Job drawing, mm, ordinate dimensions from the low corner. One solid piece. Give positions to 0.01 mm unless a question says otherwise; leave off trailing zeros. Order: outer loops, then holes, each group sorted by start corner. A loop starts at its lowest first (then second) coordinate and runs counter-clockwise, first axis right, second up. Notation, with made-up numbers: (43, 68) -> (92, 68) arc R6 ccw to (92, 74) -> close; hole circle Ø10 at (37.5, 41). An arc over 180 degrees is marked (long way). Write item = value, one per line. Start each with the question number.
(1) Flat gauge pins, fed straight in: pin 1 (4 mm diameter, centred on x = 27, y = 51.875, fed in from -Z); pin 2 (1.5 mm diameter, centred on x = 12, z = 1.5, fed in from -Y); pin 3 (2.5 mm diameter, centred on x = 51.875, y = 27, fed in from -Z); pin 4 (1 mm diameter, centred on x = 6, z = 4.5, fed in from -Y). Where does each tip first touch, or does it go through?
(2) Saw through at A-A, the plane x = 27. List the corners of the cut face in (y, z) (3 decimals).
(3) Two-plate mould, pull along Y, no slides. Class the marked faces 1, 2 and 3: pulls with the +Y half, pulls with the -Y half, needs draft (parallel to the pull), parting line crosses it, or undercut.
(4) Probe line 1 along Y through (x, z) = (27, 5) (3 decimals); line 2 along X through (y, z) = (17, 8.5); line 3 along X through (y, z) = (20, 8). List the from-to ranges inside material, lowest first. Write a range as from..to.
(5) Saw through at B-B, the plane z = 4.5. List the corners of the cut face in (x, y) (3 decimals), then the cut area to 3 significant figures.
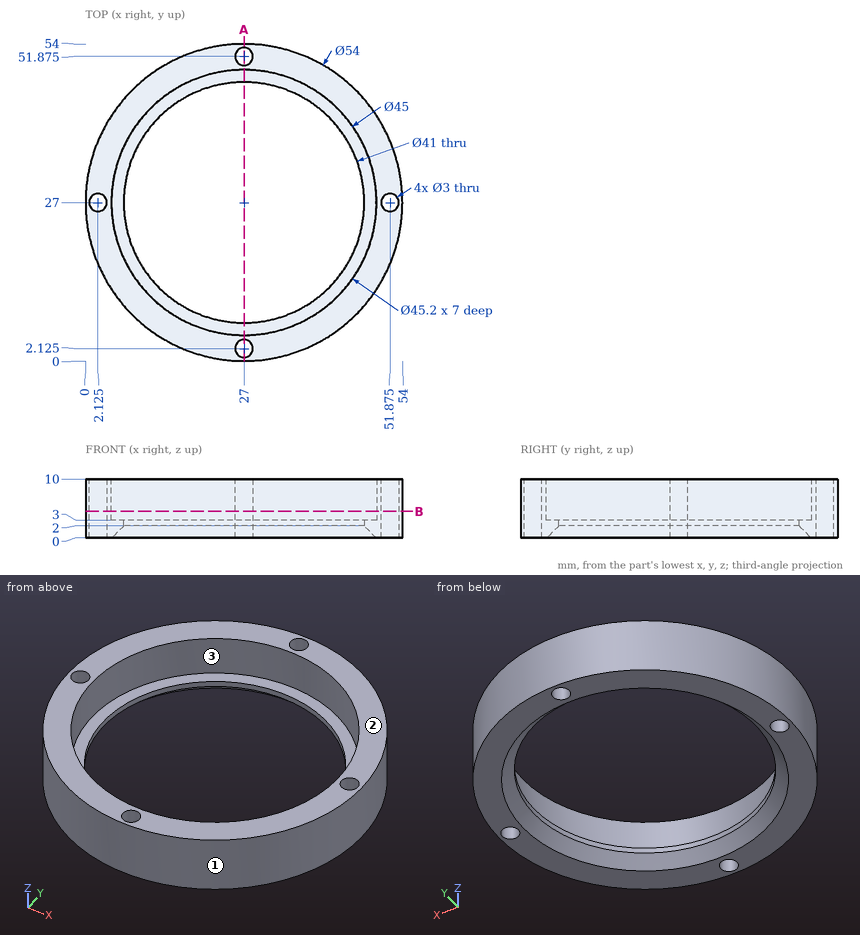
Results list:
q1.pin_1 = 0
q1.pin_2 = 4.07
q1.pin_3 = through
q1.pin_4 = 9.43
q2.outline = (0, 0) -> (0.625, 0) -> (0.625, 10) -> (0, 10) -> close; (3.625, 0) -> (4.5, 0) -> (6.5, 2) -> (6.5, 3) -> (4.4, 3) -> (4.4, 10) -> (3.625, 10) -> close; (47.5, 2) -> (49.5, 0) -> (50.375, 0) -> (50.375, 10) -> (49.6, 10) -> (49.6, 3) -> (47.5, 3) -> close; (53.375, 0) -> (54, 0) -> (54, 10) -> (53.375, 10) -> close
q3.face_1 = parting line crosses it
q3.face_2 = needs draft
q3.face_3 = undercut
q4.line_1 = 0..0.625, 3.625..4.4, 49.6..50.375, 53.375..54
q4.line_2 = 1.92..6.73, 47.27..52.08
q4.line_3 = 0.92..5.51, 48.49..53.08
q5.outline = circle Ø54 at (27, 27); hole circle Ø3 at (2.125, 27); hole circle Ø45.2 at (27, 27); hole circle Ø3 at (27, 2.125); hole circle Ø3 at (27, 51.875); hole circle Ø3 at (51.875, 27)
q5.area = 657 mm^2
